```python
from build123d import *

# Parameters (mm, degrees)
SKETCH1_R           = 1.450000001
BOSS_EXTRUDE1_DEPTH = 10


with BuildPart() as part:
    # Sketch1 → Boss-Extrude1 (new body)
    with BuildSketch(Plane.XY):
        with BuildLine():
            Line((-13.21790593, 0.411052326), (-17.105565361, -0.61539898))
            Line((-17.105565361, -0.61539898), (-20.954961557, -1.631747717))
            ThreePointArc((-20.954961557, -1.631747717), (-22.49079308, -1.415225897), (-23.410010994, -0.165946667))
            ThreePointArc((-23.410010994, -0.165946667), (105.268891372, 51.211716755), (-3.564921525, -34.53864991))
            ThreePointArc((-3.564921525, -34.53864991), (-4.187220117, -33.11794423), (-3.606817752, -31.679614205))
            Line((-3.606817752, -31.679614205), (-0.801935828, -28.854113678))
            Line((-0.801935828, -28.854113678), (2.030826794, -26.000527503))
            ThreePointArc((2.030826794, -26.000527503), (3.417973795, -25.409812538), (4.823439838, -25.955510416))
            ThreePointArc((4.823439838, -25.955510416), (94.876586526, 45.211716755), (-11.782613467, 2.807017621))
            ThreePointArc((-11.782613467, 2.807017621), (-12.012758263, 1.316999385), (-13.21790593, 0.411052326))
        make_face()
        with Locations((-17.172139776, 32.776135645)):
            Circle(SKETCH1_R, mode=Mode.SUBTRACT)
        with Locations((-10.778512735, 48.211716758)):
            Circle(SKETCH1_R, mode=Mode.SUBTRACT)
        with Locations((-19.352886894, 16.211716758)):
            Circle(SKETCH1_R, mode=Mode.SUBTRACT)
        with Locations((106.466365989, -0.352702128)):
            Circle(SKETCH1_R, mode=Mode.SUBTRACT)
        with Locations((100.07273895, -15.788283242)):
            Circle(SKETCH1_R, mode=Mode.SUBTRACT)
        with Locations((89.901947104, -29.043117238)):
            Circle(SKETCH1_R, mode=Mode.SUBTRACT)
        with Locations((76.647113107, -39.213909086)):
            Circle(SKETCH1_R, mode=Mode.SUBTRACT)
        with Locations((61.211531993, -45.607536126)):
            Circle(SKETCH1_R, mode=Mode.SUBTRACT)
        with Locations((44.647113106, -47.788283244)):
            Circle(SKETCH1_R, mode=Mode.SUBTRACT)
        with Locations((28.082694219, -45.607536126)):
            Circle(SKETCH1_R, mode=Mode.SUBTRACT)
        with Locations((12.647113106, -39.213909086)):
            Circle(SKETCH1_R, mode=Mode.SUBTRACT)
        with Locations((-0.607720889, 61.466550753)):
            Circle(SKETCH1_R, mode=Mode.SUBTRACT)
        with Locations((12.647113108, 71.637342599)):
            Circle(SKETCH1_R, mode=Mode.SUBTRACT)
        with Locations((28.08269422, 78.030969639)):
            Circle(SKETCH1_R, mode=Mode.SUBTRACT)
        with Locations((44.647113106, 80.211716756)):
            Circle(SKETCH1_R, mode=Mode.SUBTRACT)
        with Locations((61.211531992, 78.030969639)):
            Circle(SKETCH1_R, mode=Mode.SUBTRACT)
        with Locations((76.647113105, 71.637342599)):
            Circle(SKETCH1_R, mode=Mode.SUBTRACT)
        with Locations((89.901947102, 61.466550752)):
            Circle(SKETCH1_R, mode=Mode.SUBTRACT)
        with Locations((100.072738948, 48.211716757)):
            Circle(SKETCH1_R, mode=Mode.SUBTRACT)
        with Locations((106.466365989, 32.776135644)):
            Circle(SKETCH1_R, mode=Mode.SUBTRACT)
        with Locations((108.647113106, 16.211716758)):
            Circle(SKETCH1_R, mode=Mode.SUBTRACT)
    extrude(amount=BOSS_EXTRUDE1_DEPTH)


solid = part.part
```
CAD build for the part. Positions are in the model's coordinates, mm. Round coordinates to 2 decimals unless told otherwise and drop trailing zeros. Order: outer loops, then holes, each group sorted by start corner. A loop starts at its lowest first (then second) coordinate and runs counter-clockwise, first axis right, second up. Notation, with made-up numbers: (89, 88.5) - (96, 88.5) arc R18 ccw to (96, 118.5) - close; hole circle Ø7 at (-21.5, -39.5). An arc over 180 degrees is marked (long way). Use CSV: the item, a comma, the result in double quotes. Start each with the question number.
1) Pin check, flat tips, straight feed: pin 1 Ø5 at (x, z) = (46.5, 2) entering from -Y; pin 2 Ø1 at (y, z) = (56, 5) entering from +X; pin 3 Ø2.5 at (x, y) = (-0.61, 61.47) entering from +Z; pin 4 Ø2 at (y, z) = (48, 2) entering from -X. Stop position of each tip, or through.
2) Two-plate mould, pull along Y, no slides. Class faces 1 (the cylindrical face through (103.82, 53.61, 4.93)), 2 (the cylindrical face through (95.994, 43.184, 4.93)), 3 (the flat face through (102, 27, 0)): pulls with the +Y half, pulls with the -Y half, needs draft (parallel to the pull), parting line crosses it, or undercut.
3) Wall check: L1, parallel to X at y = 16.5, z = 9.25; L2, parallel to Y at x = 12.5, z = 8.25; L3, parallel to Y at x = 76, z = 9. Give the ranges that are in metal, low to high. Write a range as [from, to].
4) Saw through at B-B (y = 7). List the corners of the cut face in (x, z), and give its area (3 significant figures).
5) Saw through at C-C (z = 3.75). Count the separate pieces of the cut face and the enclosed holes in it, and give its area (3 significant figures).
6) Saw through at A-A (x = 36). List the corners of the cut face in (y, z), and give its area (3 significant figures).
Values follow:
1,pin 1,"stops at y = -53.79"
1,pin 2,"stops at x = 102.58"
1,pin 3,"passes through"
1,pin 4,"stops at x = -18.22"
2,face 1,"parting line crosses it"
2,face 2,"undercut"
2,face 3,"needs draft"
3,L1,"x = [-25.35, -20.77], [-17.93, -13.35], [102.65, 107.23], [110.07, 114.65]"
3,L2,"y = [-45.97, -40.66], [-37.77, -32.06], [64.49, 70.19], [73.08, 78.39]"
3,L3,"y = [-46.37, -40.51], [-37.92, -32.58], [65.01, 70.34], [72.93, 78.8]"
4,outline,"(-24.74, 0) - (-12.62, 0) - (-12.62, 10) - (-24.74, 10) - close; (101.91, 0) - (114.04, 0) - (114.04, 10) - (101.91, 10) - close"
4,area,"243 mm2"
5,separate pieces,"1"
5,enclosed holes,"21"
5,area,"4,290 mm2"
6,outline,"(-53.25, 0) - (-41.14, 0) - (-41.14, 10) - (-53.25, 10) - close; (73.56, 0) - (85.68, 0) - (85.68, 10) - (73.56, 10) - close"
6,area,"242 mm2"
